Source: CAD feature listing. Evaluate the final solid. Frame: model axes, mm. A direction names the side the tool comes from. Give positions to 0.01 mm unless a question says otherwise; leave off trailing zeros. Order: outer loops, then holes, each group sorted by start corner. A loop starts at its lowest first (then second) coordinate and runs counter-clockwise, first axis right, second up. Notation, with made-up numbers: (-13.5, 6) - (44.5, 6) arc R22 ccw to (44.5, 18) - close; hole circle Ø11 at (50, -11). An arc over 180 degrees is marked (long way). Write each question's results on one line, items separated by ' | '. Start each with the question number.
Item 1: Mould query, pull axis X, two halves, no side actions, for faces 4 (the flat face through (8, -12, -12)), 5 (the cylindrical face through (10.859, -14.797, 0.986)), 6 (the cylindrical face through (12.77, -10.5, 0.03)). Classes: released by +X, released by -X, zero draft, split by the parting line, or undercut.
Item 2: Section C-C on z = -6.5. Output: boundary loops of the cut face in (x, y), and give its area (3 significant figures).
Item 3: Section A-A on y = -13.5. Output: boundary loops of the cut face in (x, z).
Item 4: Section D-D on y = -15.75. Output: boundary loops of the cut face in (x, z), and give its area (3 significant figures).
Item 5: Line query: line 1 along Y through (x, z) = (8, 1.7); line 2 along Z through (x, y) = (10, -7.5); line 3 along Y through (x, z) = (6.25, 1). Output: solid intervals per line, ascending.
Item 6: Contact query for flat-ended pins moving along their axis: pin 1 Ø1.5 at (x, z) = (11.5, 0.5) entering from -Y; pin 2 Ø1 at (y, z) = (-12, -4) entering from -X; pin 3 Ø1.5 at (x, z) = (11, -1.5) entering from -Y. Output: stop coordinate, or through.
Item 7: Set-up query: faces 1 (the cylindrical face through (6.526, -13.352, -6.93)), 2 (the flat face through (7.9, -10.8, 2)), 3 (the cylindrical face through (5.141, -9.203, 0.986)). Return all of +Z, -Z, +X, -X, +Y, -Y with unobstructed straight access to the full face (end or side cutting, diameter ignored); none if empty.
Item 8: Section B-B on x = 5.75. Output: boundary loops of the cut face in (y, z), and give its area (3 significant figures).
```python
from build123d import *

# Parameters (mm, degrees)
F0_R     = 5
F0_R_2   = 1.5
F1_DEPTH = 2
F2_DEPTH = 2
F3_DEPTH = 2
F4_R     = 2
F4_R_2   = 1.5
F5_DEPTH = 10
F6_R     = 1
F7_DEPTH = 0.5


with BuildPart() as f1:
    # F0 (on Top) → F1 (new body)
    with BuildSketch(Plane.XY):
        with Locations((8, -12)):
            Circle(F0_R)
        with BuildLine():
            ThreePointArc((12, -12), (10.8284271247, -14.8284271247), (8, -16))
            ThreePointArc((8, -16), (7.2362373842, -15.6454972244), (7.0139867028, -14.8333333333))
            ThreePointArc((7.0139867028, -14.8333333333), (7.3545027756, -14.2362373842), (8, -14))
            ThreePointArc((8, -14), (9.4142135624, -13.4142135624), (10, -12))
            ThreePointArc((10, -12), (10.2362373842, -11.3545027756), (10.8333333333, -11.0139867028))
            ThreePointArc((10.8333333333, -11.0139867028), (11.6454972244, -11.2362373842), (12, -12))
        make_face(mode=Mode.SUBTRACT)
        with BuildLine():
            ThreePointArc((8, -10), (6.5857864376, -10.5857864376), (6, -12))
            ThreePointArc((6, -12), (5.7637626158, -12.6454972244), (5.1666666667, -12.9860132972))
            ThreePointArc((5.1666666667, -12.9860132972), (4.3545027756, -12.7637626158), (4, -12))
            ThreePointArc((4, -12), (5.1715728753, -9.1715728753), (8, -8))
            ThreePointArc((8, -8), (8.7071067812, -8.2928932188), (9, -9))
            ThreePointArc((9, -9), (8.9964971895, -9.0836262603), (8.9860132972, -9.1666666667))
            ThreePointArc((8.9860132972, -9.1666666667), (8.6454972244, -9.7637626158), (8, -10))
        make_face(mode=Mode.SUBTRACT)
        with Locations((8, -12)):
            Circle(F0_R_2, mode=Mode.SUBTRACT)
        with Locations((8, -12)):
            Circle(F0_R_2)
    extrude(amount=F1_DEPTH)

    # F0 (on Top) → F2 (join)
    with BuildSketch(Plane.XY):
        with Locations((8, -12)):
            Circle(F0_R)
        with BuildLine():
            ThreePointArc((12, -12), (10.8284271247, -14.8284271247), (8, -16))
            ThreePointArc((8, -16), (7.2362373842, -15.6454972244), (7.0139867028, -14.8333333333))
            ThreePointArc((7.0139867028, -14.8333333333), (7.3545027756, -14.2362373842), (8, -14))
            ThreePointArc((8, -14), (9.4142135624, -13.4142135624), (10, -12))
            ThreePointArc((10, -12), (10.2362373842, -11.3545027756), (10.8333333333, -11.0139867028))
            ThreePointArc((10.8333333333, -11.0139867028), (11.6454972244, -11.2362373842), (12, -12))
        make_face(mode=Mode.SUBTRACT)
        with BuildLine():
            ThreePointArc((8, -10), (6.5857864376, -10.5857864376), (6, -12))
            ThreePointArc((6, -12), (5.7637626158, -12.6454972244), (5.1666666667, -12.9860132972))
            ThreePointArc((5.1666666667, -12.9860132972), (4.3545027756, -12.7637626158), (4, -12))
            ThreePointArc((4, -12), (5.1715728753, -9.1715728753), (8, -8))
            ThreePointArc((8, -8), (8.7071067812, -8.2928932188), (9, -9))
            ThreePointArc((9, -9), (8.9964971895, -9.0836262603), (8.9860132972, -9.1666666667))
            ThreePointArc((8.9860132972, -9.1666666667), (8.6454972244, -9.7637626158), (8, -10))
        make_face(mode=Mode.SUBTRACT)
        with Locations((8, -12)):
            Circle(F0_R_2, mode=Mode.SUBTRACT)
        with BuildLine():
            ThreePointArc((9, -15), (8.7071067812, -15.7071067812), (8, -16))
            ThreePointArc((8, -16), (10.8284271247, -14.8284271247), (12, -12))
            ThreePointArc((12, -12), (11.6454972244, -12.7637626158), (10.8333333333, -12.9860132972))
            ThreePointArc((10.8333333333, -12.9860132972), (10.1213203436, -14.1213203436), (8.9860132972, -14.8333333333))
            ThreePointArc((8.9860132972, -14.8333333333), (8.9964971895, -14.9163737397), (9, -15))
        make_face()
        with BuildLine():
            ThreePointArc((8.9860132972, -14.8333333333), (10.1213203436, -14.1213203436), (10.8333333333, -12.9860132972))
            ThreePointArc((10.8333333333, -12.9860132972), (10.2362373842, -12.6454972244), (10, -12))
            ThreePointArc((10, -12), (9.4142135624, -13.4142135624), (8, -14))
            ThreePointArc((8, -14), (8.6454972244, -14.2362373842), (8.9860132972, -14.8333333333))
        make_face()
        with BuildLine():
            ThreePointArc((10.8333333333, -12.9860132972), (11.6454972244, -12.7637626158), (12, -12))
            ThreePointArc((12, -12), (11.6454972244, -11.2362373842), (10.8333333333, -11.0139867028))
            ThreePointArc((10.8333333333, -11.0139867028), (11, -12), (10.8333333333, -12.9860132972))
        make_face()
        with BuildLine():
            ThreePointArc((10.8333333333, -12.9860132972), (11, -12), (10.8333333333, -11.0139867028))
            ThreePointArc((10.8333333333, -11.0139867028), (10.2362373842, -11.3545027756), (10, -12))
            ThreePointArc((10, -12), (10.2362373842, -12.6454972244), (10.8333333333, -12.9860132972))
        make_face()
        with BuildLine():
            ThreePointArc((8, -14), (7.3545027756, -14.2362373842), (7.0139867028, -14.8333333333))
            ThreePointArc((7.0139867028, -14.8333333333), (8, -15), (8.9860132972, -14.8333333333))
            ThreePointArc((8.9860132972, -14.8333333333), (8.6454972244, -14.2362373842), (8, -14))
        make_face()
        with BuildLine():
            ThreePointArc((7.0139867028, -14.8333333333), (7.2362373842, -15.6454972244), (8, -16))
            ThreePointArc((8, -16), (8.7071067812, -15.7071067812), (9, -15))
            ThreePointArc((9, -15), (8.9964971895, -14.9163737397), (8.9860132972, -14.8333333333))
            ThreePointArc((8.9860132972, -14.8333333333), (8, -15), (7.0139867028, -14.8333333333))
        make_face()
        with BuildLine():
            ThreePointArc((7.0139867028, -9.1666666667), (7.3545027756, -9.7637626158), (8, -10))
            ThreePointArc((8, -10), (8.6454972244, -9.7637626158), (8.9860132972, -9.1666666667))
            ThreePointArc((8.9860132972, -9.1666666667), (8, -9), (7.0139867028, -9.1666666667))
        make_face()
        with BuildLine():
            ThreePointArc((8, -8), (7.2362373842, -8.3545027756), (7.0139867028, -9.1666666667))
            ThreePointArc((7.0139867028, -9.1666666667), (8, -9), (8.9860132972, -9.1666666667))
            ThreePointArc((8.9860132972, -9.1666666667), (8.9964971895, -9.0836262603), (9, -9))
            ThreePointArc((9, -9), (8.7071067812, -8.2928932188), (8, -8))
        make_face()
        with BuildLine():
            ThreePointArc((5.1666666667, -11.0139867028), (5.7637626158, -11.3545027756), (6, -12))
            ThreePointArc((6, -12), (6.5857864376, -10.5857864376), (8, -10))
            ThreePointArc((8, -10), (7.3545027756, -9.7637626158), (7.0139867028, -9.1666666667))
            ThreePointArc((7.0139867028, -9.1666666667), (7.2362373842, -8.3545027756), (8, -8))
            ThreePointArc((8, -8), (5.1715728753, -9.1715728753), (4, -12))
            ThreePointArc((4, -12), (4.3545027756, -11.2362373842), (5.1666666667, -11.0139867028))
        make_face()
        with BuildLine():
            ThreePointArc((5.1666666667, -12.9860132972), (5.7637626158, -12.6454972244), (6, -12))
            ThreePointArc((6, -12), (5.7637626158, -11.3545027756), (5.1666666667, -11.0139867028))
            ThreePointArc((5.1666666667, -11.0139867028), (5, -12), (5.1666666667, -12.9860132972))
        make_face()
        with BuildLine():
            ThreePointArc((5.1666666667, -12.9860132972), (5, -12), (5.1666666667, -11.0139867028))
            ThreePointArc((5.1666666667, -11.0139867028), (4.3545027756, -11.2362373842), (4, -12))
            ThreePointArc((4, -12), (4.3545027756, -12.7637626158), (5.1666666667, -12.9860132972))
        make_face()
    extrude(amount=-F2_DEPTH)

    # F0 (on Top) → F3 (join)
    with BuildSketch(Plane.XY):
        with Locations((8, -12)):
            Circle(F0_R_2)
    extrude(amount=-F3_DEPTH)

    # F4 (on face) → F5 (join)
    with BuildSketch(Plane(origin=(0, 0, -2), x_dir=(1, 0, 0), z_dir=(0, 0, -1))):
        with Locations((8, 12)):
            Circle(F4_R)
        with Locations((8, 12)):
            Circle(F4_R_2, mode=Mode.SUBTRACT)
        with Locations((8, 12)):
            Circle(F4_R_2)
    extrude(amount=F5_DEPTH)

    # F6 (on face) → F7 (cut)
    with BuildSketch(Plane.XY.offset(2)):
        with Locations((8, -12)):
            Circle(F6_R)
    extrude(amount=-F7_DEPTH, mode=Mode.SUBTRACT)


solid = f1.part
```
Evaluation:
1) face 4: zero draft | face 5: undercut | face 6: split by the parting line
2) outline: circle Ø4 at (8, -12) | area: 12.6 mm^2
3) outline: (3.23, -2) - (6.68, -2) - (6.68, -12) - (9.32, -12) - (9.32, -2) - (12.77, -2) - (12.77, 2) - (11.71, 2) - (11.71, 0) - (9.32, 0) - (9.32, 2) - (3.23, 2) - close
4) outline: (4.69, -2) - (11.31, -2) - (11.31, 2) - (9.39, 2) - (9.39, 0) - (7.34, 0) - (7.34, 2) - (4.69, 2) - close | area: 22.4 mm^2
5) line 1: y = -17 to -16, -14 to -13, -11 to -10, -8 to -7 | line 2: z = -2 to 2 | line 3: y = -16.68 to -11.03, -8.4 to -7.32
6) pin 1: stops at y = -16.18 | pin 2: stops at x = 6 | pin 3: stops at y = -16.47
7) face 1: -Z | face 2: +Z, +X, -X, +Y, -Y | face 3: +Z
8) outline: (-16.47, -2) - (-7.53, -2) - (-7.53, 2) - (-8.69, 2) - (-8.69, 0) - (-12.66, 0) - (-12.66, 2) - (-16.47, 2) - close | area: 27.8 mm^2
